The listing builds one solid part. Answer for the finished solid, in the listing's coordinates (mm). Face numbers are marked on the shaded views. Give positions to 0.01 mm unless a question says otherwise; leave off trailing zeros. Write each loop counter-clockwise with the first axis right and the second up, starting at its lowest first coordinate (ties: lowest second). Pieces come first, ordered by that corner, then holes. Notation, with made-up numbers: (18, 45.25) - (56, 45.25) arc R26 ccw to (56, 68.25) - close; hole circle Ø8 at (-14.5, 50). An arc over 180 degrees is marked (long way). Write each question's results on one line, items separated by ' | '. Start each with the question number.
Q1. For a pull along Z with two mould halves and no side action, classify the marked faces 1, 2 and 3 as pulls with the +Z half, pulls with the -Z half, needs draft (parallel to the pull), parting line crosses it, or undercut.
Q2. Section C-C (x = 2) is taken. Determine the outline of the cut face in (y, z).
Q3. Flat-ended cylindrical pins translate along their axes: pin 1 Ø1.9 at (x, y) = (-22, -64.16) entering from -Z; pin 2 Ø5 at (x, y) = (-3, -40.5) entering from +Z; pin 3 Ø5 at (x, z) = (10, -25.5) entering from -Y; pin 4 Ø2 at (x, z) = (-14, 53) entering from -Y. Find the tip coordinate at first contact, or state that the pin passes through.
Q4. Section B-B (y = -17) is taken. Determine the outline of the cut face in (x, z) (3 decimals), plus the area to 3 significant figures.
Q5. Section A-A (x = 22) is taken. Determine the outline of the cut face in (y, z).
Q6. Section D-D (z = -37.5) is taken. Determine the outline of the cut face in (x, y) (3 decimals).
Q7. Find the intervals of material crossed by probe 1 along X at (y, z) = (-64, -52) (3 decimals); probe 2 along Y at (x, z) = (-22, -52.2); probe 3 along Y at (x, z) = (22, -52.55), in increasing order.
```python
from build123d import *

# Parameters (mm, degrees)
SKETCH1_W                = 68.85
SKETCH1_H                = 107
BOSS_EXTRUDE1_DEPTH      = 2
SKETCH2_W                = 68.85
SKETCH2_H                = 2
BOSS_EXTRUDE2_DEPTH      = 67
CUT_EXTRUDE2_REACH       = 132.855
SKETCH5_W                = 68.85
SKETCH5_H                = 2
BOSS_EXTRUDE3_DEPTH      = 51
SKETCH6_W                = 68.85
SKETCH6_H                = 2
BOSS_EXTRUDE4_DEPTH      = 20.36
BOSS_EXTRUDE5_DEPTH      = 1.5
SKETCH13_W               = 2
SKETCH13_H               = 1.5
BOSS_EXTRUDE8_DEPTH      = 3
CUT_EXTRUDE4_REACH       = 97.75
SKETCH9_R                = 1.75
FILLET1_R                = 1.5
FILLET2_R                = 3
FILLET3_R                = 1.5
FILLET4_R                = 3
CUT_EXTRUDE5_REACH       = 111.975
SKETCH10_R               = 1.75
CHAMFER1_SIZE            = 2
SKETCH11_W               = 2
SKETCH11_H               = 109
BOSS_EXTRUDE6_DEPTH      = 4.5
SKETCH14_W               = 68.85
SKETCH14_H               = 0.5
BOSS_EXTRUDE9_DEPTH      = 2
FILLET5_R                = 2
FILLET6_R                = 4
FILLET8_R                = 4
CUT_EXTRUDE6_DEPTH       = 1
CUT_EXTRUDE7_DEPTH       = 125.986967721
SKETCH17_W               = 68.85
SKETCH17_H               = 2
BOSS_EXTRUDE10_DEPTH     = 8.66
SKETCH18_W               = 2
SKETCH18_H               = 68.16
BOSS_EXTRUDE11_DEPTH     = 2
SKETCH19_W               = 2
SKETCH19_H               = 68.16
BOSS_EXTRUDE12_DEPTH     = 2
FILLET9_R                = 4
FILLET10_R               = 4
FILLET11_R               = 1.5
BOSS_EXTRUDE13_START     = -2
BOSS_EXTRUDE13_OUTLINE_R = 1.6
BOSS_EXTRUDE13_DEPTH     = 2
BOSS_EXTRUDE14_START     = 15
SKETCH21_W               = 7.5
SKETCH21_H               = 1.5
BOSS_EXTRUDE14_DEPTH     = 4
CHAMFER2_SIZE            = 0.5
CHAMFER3_SIZE            = 0.75


# Read off the part's stored shape, not the designer's step: Boss-Extrude13
with BuildPart() as part:
    # Sketch1 → Boss-Extrude1 (new body)
    with BuildSketch(Plane(origin=(0, 0, 0), x_dir=(1, 0, 0), z_dir=(0, 1, 0))):
        Rectangle(SKETCH1_W, SKETCH1_H)
    extrude(amount=BOSS_EXTRUDE1_DEPTH)

    # Sketch2 → Boss-Extrude2 (add)
    with BuildSketch(Plane.XZ):
        with Locations((0, -52.5)):
            Rectangle(SKETCH2_W, SKETCH2_H)
    extrude(amount=BOSS_EXTRUDE2_DEPTH)

    # Sketch4 → Cut-Extrude2 (cut, up to next)
    with BuildSketch(Plane(origin=(0, 0, -53.5), x_dir=(-1, 0, 0), z_dir=(0, 0, -1)), mode=Mode.PRIVATE) as cut_extrude2_sk1:
        Polygon((-6.85, -15.65), (-6.85, -20.95), (-5.325, -20.95), (6.85, -20.95), (6.85, -15.65), (25.15, -15.65), (25.15, -35.75), (-25.15, -35.75), (-25.15, -15.65), align=None)
    cut_extrude2_tool1 = extrude(cut_extrude2_sk1.sketch, amount=-CUT_EXTRUDE2_REACH, mode=Mode.PRIVATE) & part.part
    add(cut_extrude2_tool1.solids().sort_by_distance((0, -26.272573, -53.5))[0], mode=Mode.SUBTRACT)

    # Sketch5 → Boss-Extrude3 (add)
    with BuildSketch(Plane.XY.offset(-51.5)):
        with Locations((0, -66)):
            Rectangle(SKETCH5_W, SKETCH5_H)
    extrude(amount=BOSS_EXTRUDE3_DEPTH)

    # Sketch6 → Boss-Extrude4 (add)
    with BuildSketch(Plane.XZ.offset(67)):
        with Locations((0, -1.5)):
            Rectangle(SKETCH6_W, SKETCH6_H)
    extrude(amount=BOSS_EXTRUDE4_DEPTH)

    # Sketch8 → Boss-Extrude5 (add)
    with BuildSketch(Plane(origin=(0, 2, 0), x_dir=(1, 0, 0), z_dir=(0, 1, 0))):
        Polygon((-36.425, 50.5), (-34.425, 50.5), (-34.425, -53.5), (34.425, -53.5), (34.425, 50.5), (36.425, 50.5), (36.425, -55.5), (-36.425, -55.5), align=None)
    extrude(amount=-BOSS_EXTRUDE5_DEPTH)

    # Sketch13 → Boss-Extrude8 (add)
    with BuildSketch(Plane(origin=(0, 0, -50.5), x_dir=(-1, 0, 0), z_dir=(0, 0, -1))):
        with Locations((35.425, 1.25)):
            Rectangle(SKETCH13_W, SKETCH13_H)
        with Locations((-35.425, 1.25)):
            Rectangle(SKETCH13_W, SKETCH13_H)
    extrude(amount=BOSS_EXTRUDE8_DEPTH)

    # Sketch9 → Cut-Extrude4 (cut, up to next)
    with BuildSketch(Plane.XZ.offset(67), mode=Mode.PRIVATE) as cut_extrude4_sk1:
        with Locations(Location((-25, -23.48, 0), (0, 0, 270))):
            Circle(SKETCH9_R)
    cut_extrude4_tool1 = extrude(cut_extrude4_sk1.sketch, amount=-CUT_EXTRUDE4_REACH, mode=Mode.PRIVATE) & part.part
    # Sketch9 → Cut-Extrude4 (cut, up to next)
    with BuildSketch(Plane.XZ.offset(67), mode=Mode.PRIVATE) as cut_extrude4_sk2:
        with Locations(Location((25, -23.48, 0), (0, 0, 270))):
            Circle(SKETCH9_R)
    cut_extrude4_tool2 = extrude(cut_extrude4_sk2.sketch, amount=-CUT_EXTRUDE4_REACH, mode=Mode.PRIVATE) & part.part
    add(cut_extrude4_tool1.solids().sort_by_distance((-25, -67, -23.48))[0], mode=Mode.SUBTRACT)
    add(cut_extrude4_tool2.solids().sort_by_distance((25, -67, -23.48))[0], mode=Mode.SUBTRACT)

    # Fillet1
    fillet1_edges = [part.edges().sort_by_distance(p)[0] for p in [
        (0, -67, -2.5),
    ]]
    fillet(fillet1_edges, radius=FILLET1_R)

    # Fillet2
    fillet2_edges = [part.edges().sort_by_distance(p)[0] for p in [
        (0, -65, -0.5),
    ]]
    fillet(fillet2_edges, radius=FILLET2_R)

    # Fillet3
    fillet3_edges = [part.edges().sort_by_distance(p)[0] for p in [
        (0, -65, -51.5),
    ]]
    fillet(fillet3_edges, radius=FILLET3_R)

    # Fillet4
    fillet4_edges = [part.edges().sort_by_distance(p)[0] for p in [
        (0, -67, -53.5),
    ]]
    fillet(fillet4_edges, radius=FILLET4_R)

    # Sketch10 → Cut-Extrude5 (cut, up to next)
    with BuildSketch(Plane.XY.offset(-0.5), mode=Mode.PRIVATE) as cut_extrude5_sk1:
        with Locations((-24.425, -79.36)):
            Circle(SKETCH10_R)
    cut_extrude5_tool1 = extrude(cut_extrude5_sk1.sketch, amount=-CUT_EXTRUDE5_REACH, mode=Mode.PRIVATE) & part.part
    # Sketch10 → Cut-Extrude5 (cut, up to next)
    with BuildSketch(Plane.XY.offset(-0.5), mode=Mode.PRIVATE) as cut_extrude5_sk2:
        with Locations((24.425, -79.36)):
            Circle(SKETCH10_R)
    cut_extrude5_tool2 = extrude(cut_extrude5_sk2.sketch, amount=-CUT_EXTRUDE5_REACH, mode=Mode.PRIVATE) & part.part
    add(cut_extrude5_tool1.solids().sort_by_distance((-24.425, -79.36, -0.5))[0], mode=Mode.SUBTRACT)
    add(cut_extrude5_tool2.solids().sort_by_distance((24.425, -79.36, -0.5))[0], mode=Mode.SUBTRACT)

    # Chamfer1
    chamfer1_edges = [part.edges().sort_by_distance(p)[0] for p in [
        (-34.425, -87.36, -1.5),
        (34.425, -87.36, -1.5),
    ]]
    chamfer(chamfer1_edges, length=CHAMFER1_SIZE)

    # Sketch11 → Boss-Extrude6 (add)
    with BuildSketch(Plane.XZ.offset(-0.5)):
        with Locations((35.425, 1)):
            Rectangle(SKETCH11_W, SKETCH11_H)
        with Locations((-35.425, 1)):
            Rectangle(SKETCH11_W, SKETCH11_H)
    extrude(amount=BOSS_EXTRUDE6_DEPTH)

    # Sketch14 → Boss-Extrude9 (add)
    with BuildSketch(Plane.XY.offset(53.5)):
        with Locations((0, 0.25)):
            Rectangle(SKETCH14_W, SKETCH14_H)
    extrude(amount=BOSS_EXTRUDE9_DEPTH)

    # Fillet5
    fillet5_edges = [part.edges().sort_by_distance(p)[0] for p in [
        (0, 0, -51.5),
        (34.425, 0, 2),
        (-34.425, 0, 2),
    ]]
    fillet(fillet5_edges, radius=FILLET5_R)

    # Fillet6
    fillet6_edges = [part.edges().sort_by_distance(p)[0] for p in [
        (0, 2, -53.5),
    ]]
    fillet(fillet6_edges, radius=FILLET6_R)

    # Fillet8
    # the kernel refuses this fillet: 4 mm, written as the material it takes off along each edge
    with BuildSketch(Plane(origin=(-36.425, 2, 65.5), x_dir=(1, 0, 0), z_dir=(0, 0, -1))) as fillet8_piece_1:
        with BuildLine():
            CenterArc((FILLET8_R, FILLET8_R), FILLET8_R, 180, 90)
            Line((0, FILLET8_R), (0, 0))
            Line((0, 0), (FILLET8_R, 0))
        make_face()
    extrude(amount=125, mode=Mode.SUBTRACT)
    with BuildSketch(Plane(origin=(36.425, 2, -59.5), x_dir=(0, -1, 0), z_dir=(0, 0, 1))) as fillet8_piece_2:
        with BuildLine():
            CenterArc((FILLET8_R, -FILLET8_R), FILLET8_R, 90, 90)
            Line((0, -FILLET8_R), (0, 0))
            Line((0, 0), (FILLET8_R, 0))
        make_face()
    extrude(amount=125, mode=Mode.SUBTRACT)

    # Sketch15 → Cut-Extrude6 (cut)
    with BuildSketch(Plane.XY.offset(55.5)):
        with BuildLine():
            Line((-36.425, -2), (-36.425, -4))
            Line((-36.425, -4), (-34.425, -4))
            Line((-34.425, -4), (-34.425, -2))
            ThreePointArc((-34.425, -2), (-33.839213562, -0.585786438), (-32.425, 0))
            Line((-32.425, 0), (32.425, 0))
            ThreePointArc((32.425, 0), (33.839213562, -0.585786438), (34.425, -2))
            Line((34.425, -2), (34.425, -4))
            Line((34.425, -4), (36.425, -4))
            Line((36.425, -4), (36.425, -2))
            ThreePointArc((36.425, -2), (35.253427125, 0.828427125), (32.425, 2))
            Line((32.425, 2), (-32.425, 2))
            ThreePointArc((-32.425, 2), (-35.253427125, 0.828427125), (-36.425, -2))
        make_face()
    extrude(amount=-CUT_EXTRUDE6_DEPTH, mode=Mode.SUBTRACT)

    # Sketch16 → Cut-Extrude7 (cut, through all)
    with BuildSketch(Plane(origin=(34.425, 0, 0), x_dir=(0, 0, -1), z_dir=(1, 0, 0))):
        with BuildLine():
            Line((2.5, -87.36), (0.5, -87.36))
            Line((0.5, -87.36), (0.5, -68))
            ThreePointArc((0.5, -68), (1.378679656, -65.878679656), (3.5, -65))
            Line((3.5, -65), (50, -65))
            ThreePointArc((50, -65), (51.060660172, -64.560660172), (51.5, -63.5))
            Line((51.5, -63.5), (53.5, -63.5))
            Line((53.5, -63.5), (53.5, -64))
            ThreePointArc((53.5, -64), (52.621320344, -66.121320344), (50.5, -67))
            Line((50.5, -67), (4, -67))
            ThreePointArc((4, -67), (2.939339828, -67.439339828), (2.5, -68.5))
            Line((2.5, -68.5), (2.5, -87.36))
        make_face()
    extrude(amount=-CUT_EXTRUDE7_DEPTH, mode=Mode.SUBTRACT)

    # Sketch17 → Boss-Extrude10 (add)
    with BuildSketch(Plane.XZ.offset(63.5)):
        with Locations((0, -52.5)):
            Rectangle(SKETCH17_W, SKETCH17_H)
    extrude(amount=BOSS_EXTRUDE10_DEPTH)

    # Sketch18 → Boss-Extrude11 (add)
    with BuildSketch(Plane(origin=(34.425, 0, 0), x_dir=(0, 0, -1), z_dir=(1, 0, 0))):
        with Locations((52.5, -38.08)):
            Rectangle(SKETCH18_W, SKETCH18_H)
    extrude(amount=BOSS_EXTRUDE11_DEPTH)

    # Sketch19 → Boss-Extrude12 (add)
    with BuildSketch(Plane.ZY.offset(34.425)):
        with Locations((-52.5, -38.08)):
            Rectangle(SKETCH19_W, SKETCH19_H)
    extrude(amount=BOSS_EXTRUDE12_DEPTH)

    # Fillet9
    fillet9_edges = [part.edges().sort_by_distance(p)[0] for p in [
        (36.425, -72.16, -52.5),
        (-36.425, -72.16, -52.5),
    ]]
    fillet(fillet9_edges, radius=FILLET9_R)

    # Fillet10
    fillet10_edges = [part.edges().sort_by_distance(p)[0] for p in [
        (35.425, -4, -51.5),
        (-35.425, -4, -51.5),
    ]]
    fillet(fillet10_edges, radius=FILLET10_R)

    # Fillet11
    fillet11_edges = [part.edges().sort_by_distance(p)[0] for p in [
        (35.425, -4, 54.5),
        (-35.425, -4, 54.5),
    ]]
    fillet(fillet11_edges, radius=FILLET11_R)

    # Boss-Extrude13 outline → Boss-Extrude13 (cut)
    with BuildSketch(Plane(origin=(0, 0, -53.5), x_dir=(-1, 0, 0), z_dir=(0, 0, -1)).offset(BOSS_EXTRUDE13_START)):
        with Locations((22, -64.16)):
            Circle(BOSS_EXTRUDE13_OUTLINE_R)
        with Locations((-22, -64.16)):
            Circle(BOSS_EXTRUDE13_OUTLINE_R)
    extrude(amount=BOSS_EXTRUDE13_DEPTH, mode=Mode.SUBTRACT)

    # Sketch21 → Boss-Extrude14 (add, symmetric)
    with BuildSketch(Plane(origin=(0, 0, 0), x_dir=(0, 0, -1), z_dir=(1, 0, 0)).offset(BOSS_EXTRUDE14_START)):
        with Locations((-52.25, -0.75)):
            Rectangle(SKETCH21_W, SKETCH21_H)
    boss_extrude14 = extrude(amount=BOSS_EXTRUDE14_DEPTH, both=True)

    # Mirror1: Boss-Extrude14 across plane
    add(boss_extrude14.mirror(Plane(origin=(0, 0, 0), x_dir=(0, 0, 1), z_dir=(1, 0, 0))))

    # Chamfer2
    chamfer2_edges = [part.edges().sort_by_distance(p)[0] for p in [
        (15, 0, 56),
        (-15, 0, 56),
    ]]
    chamfer(chamfer2_edges, length=CHAMFER2_SIZE)

    # Chamfer3
    chamfer3_edges = [part.edges().sort_by_distance(p)[0] for p in [
        (15, -1.5, 56),
        (-15, -1.5, 56),
    ]]
    chamfer(chamfer3_edges, length=CHAMFER3_SIZE)


solid = part.part
```
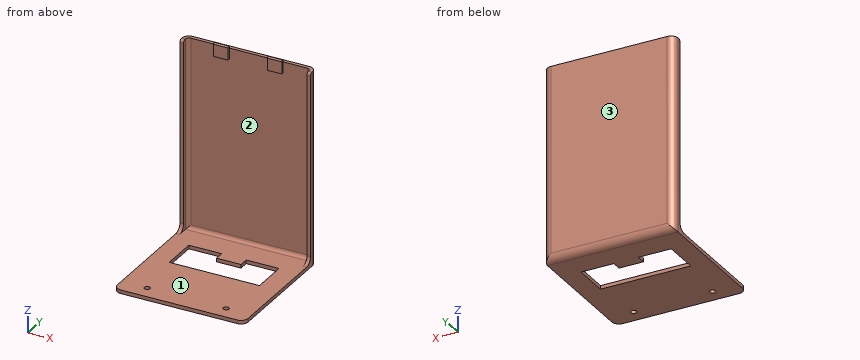
Answers below:
1) face 1: pulls with the +Z half | face 2: undercut | face 3: needs draft
2) outline: (-72.16, -53.5) - (-35.75, -53.5) - (-35.75, -51.5) - (-72.16, -51.5) - close; (-20.95, -53.5) - (-2, -53.5) arc R4 ccw to (2, -49.5) - (2, 54.5) - (0, 54.5) - (0, -49.5) arc R2 cw to (-2, -51.5) - (-20.95, -51.5) - close
3) pin 1: passes through | pin 2: stops at z = -51.5 | pin 3: stops at y = 0 | pin 4: stops at y = -1.5
4) outline: (-36.425, -53.5) - (-25.15, -53.5) - (-25.15, -51.5) - (-36.425, -51.5) - close; (-6.85, -53.5) - (6.85, -53.5) - (6.85, -51.5) - (-6.85, -51.5) - close; (25.15, -53.5) - (36.425, -53.5) - (36.425, -51.5) - (25.15, -51.5) - close | area: 72.5 mm2
5) outline: (-72.16, -53.5) - (-65.76, -53.5) - (-65.76, -51.5) - (-72.16, -51.5) - close; (-62.56, -53.5) - (-35.75, -53.5) - (-35.75, -51.5) - (-62.56, -51.5) - close; (-15.65, -53.5) - (-2, -53.5) arc R4 ccw to (2, -49.5) - (2, 54.5) - (0, 54.5) - (0, -49.5) arc R2 cw to (-2, -51.5) - (-15.65, -51.5) - close
6) outline: (-36.425, -4) - (-34.425, -4) - (-34.425, -2) arc R2 cw to (-32.425, 0) - (32.425, 0) arc R2 cw to (34.425, -2) - (34.425, -4) - (36.425, -4) - (36.425, -2) arc R4 ccw to (32.425, 2) - (-32.425, 2) arc R4 ccw to (-36.425, -2) - close
7) probe 1: x = -36.425 to -23.592, -20.408 to 20.408, 23.592 to 36.425 | probe 2: y = -72.16 to -65.76, -62.56 to -35.75, -15.65 to 0.95 | probe 3: y = -72.16 to -65.76, -62.56 to -35.75, -15.65 to 0.59
